The figure shows three views and two pictorial views of one solid part (mm, origin at its lowest corner). Answer the questions. Coordinates: 2 decimals unless noted, no trailing zeros. Loops run counter-clockwise (first coordinate to the right, second up) from the corner with the lowest first, then second, coordinate; pieces in that order, holes last. Notation, with made-up numbers: (66, -2.5) -> (73, -2.5) arc R32 ccw to (73, 33.5) -> close; hole circle Ø11 at (14.25, -13.75). An arc over 180 degrees is marked (long way). Answer in a Markdown table with one row per item.
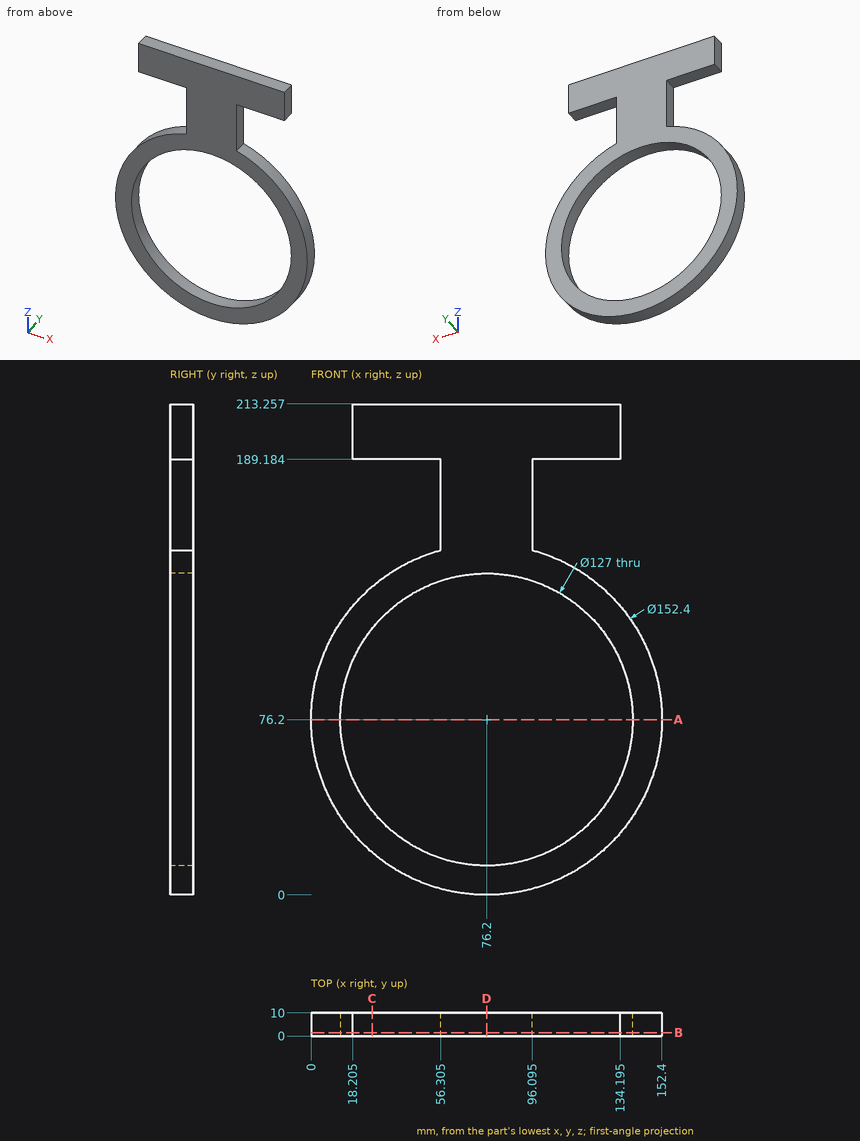
Item 1: Flat-ended cylindrical pins translate along their axes: pin 1 Ø6 at (y, z) = (8.5, 138.5) entering from +X (1 decimal); pin 2 Ø10 at (x, z) = (18, 61) entering from +Y; pin 3 Ø3 at (x, y) = (43.5, 3) entering from -Z; pin 4 Ø1 at (x, y) = (26, 6) entering from -Z. Find the tip coordinate at first contact, or state that the pin passes through.
Findings below:
| item | result |
|---|---|
| pin 1 | stops at x = 124.1 |
| pin 2 | stops at y = 10 |
| pin 3 | stops at z = 6.68 |
| pin 4 | stops at z = 18.44 |
Item 2: A cutting plane is placed at D-D, the plane x = 76.2. Determine the outline of the cut face in (y, z).
Findings below:
| item | result |
|---|---|
| outline | (0, 0) -> (10, 0) -> (10, 12.7) -> (0, 12.7) -> close; (0, 139.7) -> (10, 139.7) -> (10, 213.26) -> (0, 213.26) -> close |
Item 3: Find the intervals of material crossed by probe 1 along Z at (x, y) = (26, 8) (1 decimal); probe 2 along Z at (x, y) = (76.2, 5.5); probe 3 along X at (y, z) = (7.25, 20.5) (1 decimal), in increasing order.
Findings below:
| item | result |
|---|---|
| probe 1 | z = 18.9 to 37.3, 115.1 to 133.5, 189.2 to 213.3 |
| probe 2 | z = 0 to 12.7, 139.7 to 213.26 |
| probe 3 | x = 24.2 to 45.7, 106.7 to 128.2 |
Item 4: A cutting plane is placed at B-B, the plane y = 1.5. Determine the outline of the cut face in (x, z) (1 decimal).
Findings below:
| item | result |
|---|---|
| outline | (18.2, 189.2) -> (56.3, 189.2) -> (56.3, 149.8) arc R76.2 ccw (long way) to (96.1, 149.8) -> (96.1, 189.2) -> (134.2, 189.2) -> (134.2, 213.3) -> (18.2, 213.3) -> close; hole circle Ø127 at (76.2, 76.2) |
Item 5: A cutting plane is placed at A-A, the plane z = 76.2. Determine the outline of the cut face in (x, y), plus the area to 3 significant figures.
Findings below:
| item | result |
|---|---|
| outline | (0, 0) -> (12.7, 0) -> (12.7, 10) -> (0, 10) -> close; (139.7, 0) -> (152.4, 0) -> (152.4, 10) -> (139.7, 10) -> close |
| area | 254 mm2 |
Item 6: A cutting plane is placed at C-C, the plane x = 26.5. Determine the outline of the cut face in (y, z) (1 decimal).
Findings below:
| item | result |
|---|---|
| outline | (0, 18.4) -> (10, 18.4) -> (10, 36.7) -> (0, 36.7) -> close; (0, 115.7) -> (10, 115.7) -> (10, 134) -> (0, 134) -> close; (0, 189.2) -> (10, 189.2) -> (10, 213.3) -> (0, 213.3) -> close |
